from build123d import *

# Parameters (mm, degrees)
F0_R        = 45
F0_R_2      = 40.5
F1_DEPTH    = 10
F0_R_3      = 36.1
F2_DEPTH    = 5
F0_R_4      = 31
F3_DEPTH    = 8.4
F0_R_5      = 17.4
F4_DEPTH    = 8.4
F5_R        = 3
F1_FACE_R   = 45
F1_FACE_R_2 = 40.5
F6_DEPTH    = 5


with BuildPart() as f1:
    # F0 (on Top) → F1 (new body)
    with BuildSketch(Plane.XY):
        Circle(F0_R)
        Circle(F0_R_2, mode=Mode.SUBTRACT)
    extrude(amount=F1_DEPTH)

    # F0 (on Top) → F2 (join)
    with BuildSketch(Plane.XY):
        Circle(F0_R_2)
        Circle(F0_R_3, mode=Mode.SUBTRACT)
    extrude(amount=F2_DEPTH)

    # F0 (on Top) → F3 (join)
    with BuildSketch(Plane.XY):
        Circle(F0_R_3)
        Circle(F0_R_4, mode=Mode.SUBTRACT)
    extrude(amount=F3_DEPTH)

    # F0 (on Top) → F4 (join)
    with BuildSketch(Plane.XY):
        Circle(F0_R_4)
        Circle(F0_R_5, mode=Mode.SUBTRACT)
    extrude(amount=F4_DEPTH)

    # F5 (on face) + F1_face (on face) → F6 (join)
    with BuildSketch(Plane.XY.offset(10)):
        with BuildLine():
            ThreePointArc((66.3253242136, -9), (79.8896090165, -11.5039872942), (87.5, 0))
            ThreePointArc((87.5, 0), (79.8896090165, 11.5039872942), (66.3253242136, 9))
            Line((66.3253242136, 9), (66.3253242136, 0))
            Line((66.3253242136, 0), (66.3253242136, -9))
        make_face()
        with BuildLine():
            ThreePointArc((78, 0), (75, -3), (72, 0))
            ThreePointArc((72, 0), (75, 3), (78, 0))
        make_face(mode=Mode.SUBTRACT)
        with BuildLine():
            ThreePointArc((62.5527321378, -1.1469624085), (63.7327165773, -5.4127926501), (66.3253242136, -9))
            Line((66.3253242136, -9), (66.3253242136, 0))
            Line((66.3253242136, 0), (62.5527321378, 0))
            Line((62.5527321378, 0), (62.5527321378, -1.1469624085))
        make_face()
        with BuildLine():
            Line((66.3253242136, 0), (66.3253242136, 9))
            ThreePointArc((66.3253242136, 9), (63.7327165773, 5.4127926501), (62.5527321378, 1.1469624085))
            Line((62.5527321378, 1.1469624085), (62.5527321378, 0))
            Line((62.5527321378, 0), (66.3253242136, 0))
        make_face()
        with BuildLine():
            ThreePointArc((62.5527321378, 1.1469624085), (63.7327165773, 5.4127926501), (66.3253242136, 9))
            add(Edge.make_bspline(
                [(66.3253242136, 9), (62.5527321378, 7.0294414229), (56.1633100825, 5.6459116487), (52.2136635361, 6)],
                knots=[0, 0, 0, 0, 0.5634667873, 0.5634667873, 0.5634667873, 0.5634667873], degree=3))
            Line((52.2136635361, 6), (52.2136635361, 0))
            Line((52.2136635361, 0), (62.5, 0))
            ThreePointArc((62.5, 0), (62.5131899935, 0.5740869806), (62.5527321378, 1.1469624085))
        make_face()
        with BuildLine():
            add(Edge.make_bspline(
                [(52.2136635361, -6), (50.3742603721, -6.1649036758), (49.0640175166, -6.7066774941), (47.5582238129, -7.4185810788)],
                knots=[0.5634667873, 0.5634667873, 0.5634667873, 0.5634667873, 0.8258807981, 0.8258807981, 0.8258807981, 0.8258807981], degree=3))
            Line((52.2136635361, -6), (52.2136635361, 0))
            Line((52.2136635361, 0), (47.5582238129, 0))
            Line((47.5582238129, 0), (47.5582238129, -7.4185810788))
        make_face()
        with BuildLine():
            Line((62.5527321378, 0), (62.5527321378, 1.1469624085))
            ThreePointArc((62.5527321378, 1.1469624085), (62.5131899935, 0.5740869806), (62.5, 0))
            Line((62.5, 0), (62.5527321378, 0))
        make_face()
        with BuildLine():
            ThreePointArc((62.5, 0), (62.5131899935, -0.5740869806), (62.5527321378, -1.1469624085))
            Line((62.5527321378, -1.1469624085), (62.5527321378, 0))
            Line((62.5527321378, 0), (62.5, 0))
        make_face()
        with BuildLine():
            add(Edge.make_bspline(
                [(66.3253242136, -9), (62.5527321378, -7.0294414229), (56.1633100825, -5.6459116487), (52.2136635361, -6)],
                knots=[0, 0, 0, 0, 0.5634667873, 0.5634667873, 0.5634667873, 0.5634667873], degree=3))
            ThreePointArc((66.3253242136, -9), (63.7327165773, -5.4127926501), (62.5527321378, -1.1469624085))
            ThreePointArc((62.5527321378, -1.1469624085), (62.5131899935, -0.5740869806), (62.5, 0))
            Line((62.5, 0), (52.2136635361, 0))
            Line((52.2136635361, 0), (52.2136635361, -6))
        make_face()
        with BuildLine():
            Line((52.2136635361, 0), (52.2136635361, 6))
            add(Edge.make_bspline(
                [(52.2136635361, 6), (50.3742603721, 6.1649036758), (49.0640175166, 6.7066774941), (47.5582238129, 7.4185810788)],
                knots=[0.5634667873, 0.5634667873, 0.5634667873, 0.5634667873, 0.8258807981, 0.8258807981, 0.8258807981, 0.8258807981], degree=3))
            Line((47.5582238129, 7.4185810788), (47.5582238129, 0))
            Line((47.5582238129, 0), (52.2136635361, 0))
        make_face()
        with BuildLine():
            add(Edge.make_bspline(
                [(47.5582238129, -7.4185810788), (46.5590866207, -7.8909494696), (45.4738542162, -8.4382209279), (44.0908153701, -9)],
                knots=[0.8258807981, 0.8258807981, 0.8258807981, 0.8258807981, 1, 1, 1, 1], degree=3))
            Line((47.5582238129, -7.4185810788), (47.5582238129, 0))
            Line((47.5582238129, 0), (45, 0))
            ThreePointArc((45, 0), (44.7721268852, -4.5229032902), (44.0908153701, -9))
        make_face()
        with BuildLine():
            Line((47.5582238129, 0), (47.5582238129, 7.4185810788))
            add(Edge.make_bspline(
                [(47.5582238129, 7.4185810788), (46.5590866207, 7.8909494696), (45.4738542162, 8.4382209279), (44.0908153701, 9)],
                knots=[0.8258807981, 0.8258807981, 0.8258807981, 0.8258807981, 1, 1, 1, 1], degree=3))
            ThreePointArc((44.0908153701, 9), (44.7721268852, 4.5229032902), (45, 0))
            Line((45, 0), (47.5582238129, 0))
        make_face()
        with BuildLine():
            ThreePointArc((-44.0908153701, -9), (0, -45), (44.0908153701, -9))
            Line((44.0908153701, -9), (44.0908153701, 0))
            Line((44.0908153701, 0), (40.5, 0))
            ThreePointArc((40.5, 0), (0, -40.5), (-40.5, 0))
            Line((-40.5, 0), (-44.0908153701, 0))
            Line((-44.0908153701, 0), (-44.0908153701, -9))
        make_face()
        with BuildLine():
            Line((-51.7064335188, 0), (-51.7064335188, 6))
            add(Edge.make_bspline(
                [(-65.4197458811, 9.0034745469), (-61.6860010238, 6.9482695309), (-55.4334302889, 5.6320399313), (-51.7064335188, 6)],
                knots=[0, 0, 0, 0, 0.567027295, 0.567027295, 0.567027295, 0.567027295], degree=3))
            ThreePointArc((-65.4197458811, 9.0034745469), (-62.911579364, 5.5923771619), (-61.6860010238, 1.5396691315))
            ThreePointArc((-61.6860010238, 1.5396691315), (-61.6146344775, 0.7713043082), (-61.5908153701, 0))
            Line((-61.5908153701, 0), (-51.7064335188, 0))
        make_face()
        with BuildLine():
            ThreePointArc((-45, 0), (-44.7721268852, -4.5229032902), (-44.0908153701, -9))
            Line((-44.0908153701, -9), (-44.0908153701, 0))
            Line((-44.0908153701, 0), (-45, 0))
        make_face()
        with BuildLine():
            add(Edge.make_bspline(
                [(-65.4125331798, -8.996522563), (-61.6860010238, -6.9482695309), (-55.4331204309, -5.6323249689), (-51.7064335188, -6)],
                knots=[0, 0, 0, 0, 0.566952665, 0.566952665, 0.566952665, 0.566952665], degree=3))
            Line((-51.7064335188, -6), (-51.7064335188, 0))
            Line((-51.7064335188, 0), (-61.5908153701, 0))
            ThreePointArc((-61.5908153701, 0), (-61.6146344775, -0.7713043082), (-61.6860010238, -1.5396691315))
            ThreePointArc((-61.6860010238, -1.5396691315), (-62.9093393644, -5.5878971298), (-65.4125331798, -8.996522563))
        make_face()
        with BuildLine():
            add(Edge.make_bspline(
                [(-51.7064335188, -6), (-50.0263203675, -6.1657600088), (-48.8596569, -6.6737162451), (-47.4872474781, -7.3615768954)],
                knots=[0.566952665, 0.566952665, 0.566952665, 0.566952665, 0.8225535918, 0.8225535918, 0.8225535918, 0.8225535918], degree=3))
            Line((-47.4872474781, -7.3615768954), (-47.4872474781, 0))
            Line((-47.4872474781, 0), (-51.7064335188, 0))
            Line((-51.7064335188, 0), (-51.7064335188, -6))
        make_face()
        with BuildLine():
            ThreePointArc((-61.6860010238, 1.5396691315), (-62.911579364, 5.5923771619), (-65.4197458811, 9.0034745469))
            Line((-65.4197458811, 9.0034745469), (-65.4197458811, 0.0034745469))
            Line((-65.4197458811, 0.0034745469), (-65.4197430965, 0))
            Line((-65.4197430965, 0), (-61.6860010238, 0))
            Line((-61.6860010238, 0), (-61.6860010238, 1.5396691315))
        make_face()
        with BuildLine():
            Line((-65.4197430965, 0), (-65.4125331798, -8.996522563))
            ThreePointArc((-65.4125331798, -8.996522563), (-62.9093393644, -5.5878971298), (-61.6860010238, -1.5396691315))
            Line((-61.6860010238, -1.5396691315), (-61.6860010238, 0))
            Line((-61.6860010238, 0), (-65.4197430965, 0))
        make_face()
        with BuildLine():
            add(Edge.make_bspline(
                [(-47.4872474781, -7.3615768954), (-46.5344765882, -7.8391119468), (-45.482544702, -8.4033534464), (-44.0908153701, -9)],
                knots=[0.8225535918, 0.8225535918, 0.8225535918, 0.8225535918, 1, 1, 1, 1], degree=3))
            ThreePointArc((-44.0908153701, -9), (-44.7721268852, -4.5229032902), (-45, 0))
            Line((-45, 0), (-47.4872474781, 0))
            Line((-47.4872474781, 0), (-47.4872474781, -7.3615768954))
        make_face()
        with BuildLine():
            ThreePointArc((-45, 0), (-44.7721268852, 4.5229032902), (-44.0908153701, 9))
            add(Edge.make_bspline(
                [(-47.4872474781, 7.3617098784), (-46.5344445734, 7.8392079283), (-45.4824537219, 8.4033924504), (-44.0908153701, 9)],
                knots=[0.8225957704, 0.8225957704, 0.8225957704, 0.8225957704, 1, 1, 1, 1], degree=3))
            Line((-47.4872474781, 7.3617098784), (-47.4872474781, 0))
            Line((-47.4872474781, 0), (-45, 0))
        make_face()
        with BuildLine():
            Line((-44.0908153701, 0), (-44.0908153701, 9))
            ThreePointArc((-44.0908153701, 9), (-44.7721268852, 4.5229032902), (-45, 0))
            Line((-45, 0), (-44.0908153701, 0))
        make_face()
        with BuildLine():
            ThreePointArc((-61.6860010238, -1.5396691315), (-61.6146344775, -0.7713043082), (-61.5908153701, 0))
            Line((-61.5908153701, 0), (-61.6860010238, 0))
            Line((-61.6860010238, 0), (-61.6860010238, -1.5396691315))
        make_face()
        with BuildLine():
            ThreePointArc((-61.5908153701, 0), (-61.6146344775, 0.7713043082), (-61.6860010238, 1.5396691315))
            Line((-61.6860010238, 1.5396691315), (-61.6860010238, 0))
            Line((-61.6860010238, 0), (-61.5908153701, 0))
        make_face()
        with BuildLine():
            Line((-47.4872474781, 0), (-47.4872474781, 7.3617098784))
            add(Edge.make_bspline(
                [(-51.7064335188, 6), (-50.0266151205, 6.1658456208), (-48.8598550323, 6.6738263432), (-47.4872474781, 7.3617098784)],
                knots=[0.567027295, 0.567027295, 0.567027295, 0.567027295, 0.8225957704, 0.8225957704, 0.8225957704, 0.8225957704], degree=3))
            Line((-51.7064335188, 6), (-51.7064335188, 0))
            Line((-51.7064335188, 0), (-47.4872474781, 0))
        make_face()
        with BuildLine():
            Line((-65.4197458811, 0.0034745469), (-65.4197458811, 9.0034745469))
            ThreePointArc((-65.4197458811, 9.0034745469), (-86.5908143666, -0.0050088207), (-65.4125331798, -8.996522563))
            Line((-65.4125331798, -8.996522563), (-65.4197430965, 0))
            Line((-65.4197430965, 0), (-65.4197458811, 0.0034745469))
        make_face()
        with Locations((-74.0908153701, 0)):
            Circle(F5_R, mode=Mode.SUBTRACT)
    with BuildSketch(Plane.XY.offset(10)):
        Circle(F1_FACE_R)
        Circle(F1_FACE_R_2, mode=Mode.SUBTRACT)
    extrude(amount=-F6_DEPTH)


solid = f1.part
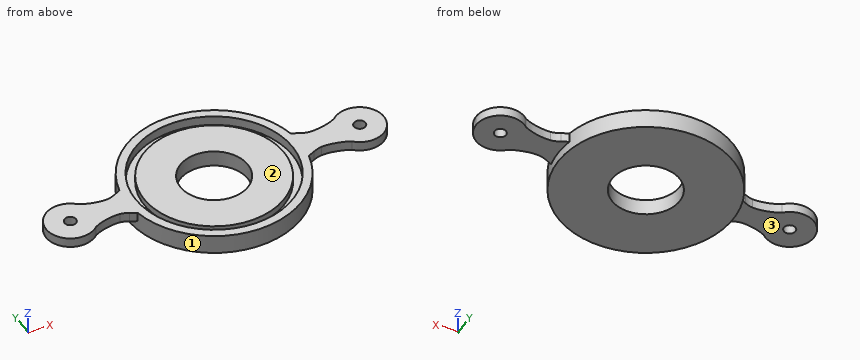
Check sheet for the modelled part. Datum: model origin and axes. Units: mm. Face numbers are marked on the shaded views. Round coordinates to 2 decimals unless told otherwise and drop trailing zeros. Loops run counter-clockwise (first coordinate to the right, second up) from the corner with the lowest first, then second, coordinate; pieces in that order, holes last. Notation, with made-up numbers: M 2.5,77.25 L 39.5,77.25 A31 cw 39.5,102.25 Z; hole C 72.5,46.5 d6. An arc over 180 degrees is marked long. One line per item, written item: value.
(1) Sectioned sample at A-A, the plane x = 75. Record the cut outline in (y, z).
Computed values:
outline: M -12.5,5 L -3,5 L -3,10 L -12.5,10 Z; M 3,5 L 12.5,5 L 12.5,10 L 3,10 Z
(2) Depth check by flat-ended pin: pin 1 Ø3 at (y, z) = (-33, 7) entering from -X; pin 2 Ø5 at (y, z) = (17.5, 7) entering from -X; pin 3 Ø7.5 at (x, y) = (-68.5, 3.5) entering from -Z. Enter the tip coordinate at first touch or a pass-through.
Computed values:
pin 1: stops at x = -32.14
pin 2: stops at x = -42.43
pin 3: stops at z = 5
(3) Thickness scan on line 1 (Y direction, x = 0, z = 8.05); line 2 (Y direction, x = 0, z = 3.75); line 3 (Y direction, x = -9, z = 6.25). Record the ranges inside material, lowest first.
Computed values:
line 1: y = -45 to -40.5, -36.1 to -17.4, 17.4 to 36.1, 40.5 to 45
line 2: y = -45 to -17.4, 17.4 to 45
line 3: y = -44.09 to -39.49, -34.96 to -14.89, 14.89 to 34.96, 39.49 to 44.09
(4) Sectioned sample at B-B, the plane y = 15. Record the cut outline in (x, z).
Computed values:
outline: M -42.43,0 L -8.82,0 L -8.82,8.4 L -32.84,8.4 L -32.84,5 L -37.62,5 L -37.62,10 L -42.43,10 Z; M 8.82,0 L 42.43,0 L 42.43,10 L 37.62,10 L 37.62,5 L 32.84,5 L 32.84,8.4 L 8.82,8.4 Z
(5) Release check for a two-part mould opening along Y. For the marked faces 1, 2 and 3 record: +Y half, -Y half, draft (parallel to the pull), parting line (faces both ways), or undercut.
Computed values:
face 1: parting line
face 2: undercut
face 3: draft
(6) Sectioned sample at C-C, the plane x = 0. Record the cut outline in (y, z), then the cut area to 3 significant figures.
Computed values:
outline: M -45,0 L -17.4,0 L -17.4,8.4 L -36.1,8.4 L -36.1,5 L -40.5,5 L -40.5,10 L -45,10 Z; M 17.4,0 L 45,0 L 45,10 L 40.5,10 L 40.5,5 L 36.1,5 L 36.1,8.4 L 17.4,8.4 Z
area: 448 mm^2
